```python
from build123d import *

# Parameters (mm, degrees)
DODANIE_WYCI_GNI_CIE1_DEPTH = 28
SZKIC2_R                    = 3
DODANIE_WYCI_GNI_CIE2_DEPTH = 6
DODANIE_WYCI_GNI_CIE3_DEPTH = 18


with BuildPart() as part:
    # Szkic1 → Dodanie-wyciągnięcie1 (new body)
    with BuildSketch(Plane.XY):
        Polygon((0, 0), (78, 0), (78, 46.489374011), (71.441538648, 49.547634765), (56.227281226, 16.920554432), (51.695742291, 19.033645741), (66.909999713, 51.660726074), (53.315382908, 58), (30, 8), (0, 8), align=None)
    extrude(amount=DODANIE_WYCI_GNI_CIE1_DEPTH)

    # Szkic2 → Dodanie-wyciągnięcie2 (add)
    with BuildSketch(Plane(origin=(31.737746535, 68.061817086, 0), x_dir=(0.9063077870366479, -0.4226182617407039, 0), z_dir=(0.4226182617407039, 0.906307787036648, 0))):
        with Locations((31.308287517, -7)):
            Circle(SZKIC2_R)
        with Locations((31.308287517, -21)):
            Circle(SZKIC2_R)
    extrude(amount=DODANIE_WYCI_GNI_CIE2_DEPTH)

    # Szkic3 → Dodanie-wyciągnięcie3 (add)
    with BuildSketch(Plane.XY):
        Polygon((0, 8), (0, 16), (24, 16), (24, 34), (42.123999112, 34), (30, 8), align=None)
    extrude(amount=DODANIE_WYCI_GNI_CIE3_DEPTH)


solid = part.part
```
Build history of the part. All positions in model axes, mm. A direction names the side the tool comes from. Round coordinates to 2 decimals unless told otherwise and drop trailing zeros. Loops run counter-clockwise (first coordinate to the right, second up) from the corner with the lowest first, then second, coordinate; pieces in that order, holes last.
Item 1: Two-plate mould, pull along X, no slides. Class faces 1 (the face through (62.61, 60.286, 20.958)), 2 (the face through (24, 25, 9)), 3 (the face through (59.359, 58.446, 4.972)): released by +X, released by -X, zero draft, split by the parting line, or undercut.
Item 2: Pin check, flat tips, straight feed: P1, Ø12, axis at y = 42.5, z = 6, coming from the -X side; P2, Ø1, axis at x = 47, z = 10.5, coming from the +Y side; P3, Ø5, axis at y = 34.5, z = 21, coming from the -X side. Stop position of each tip, or through.
Item 3: Which spindle directions (+Z, -Z, +X, -X, +Y, -Y) get a long thin tool onto all of the face, cutting with end or side? Do faces 4 (the face through (63.94, 33.46, 13.8)), 5 (the face through (48, 23, 0)), 6 (the face through (26, 18, 18)), 7 (the face through (33, 34, 9)). Say none if no direction does.
Item 4: Saw through at B-B (z = 11). List the corners of the cut face in (x, y), then the cut area to 3 significant figures.
Item 5: Saw through at A-A (y = 22.5). List the corners of the cut face in (x, z).
Item 6: Saw through at C-C (x = 23). List the corners of the cut face in (y, z).
Item 7: Drill centre lines: line 1 along Z through (x, y) = (30, 20); line 2 along Y through (x, z) = (23, 13); line 3 along Y through (x, z) = (12, 22.75). Where is each one in solid material? Low to high.
Item 8: Saw through at D-D (y = 13.5). List the corners of the cut face in (x, z), then the cut area to 3 significant figures.
Worked answers:
1. face 1: released by +X
1. face 2: released by -X
1. face 3: undercut
2. P1: stops at x = 43.29
2. P2: stops at y = 45.53
2. P3: stops at x = 41.19
3. face 4: +Z, -Z
3. face 5: -Z, +X, -X, +Y, -Y
3. face 6: +Z, -X, +Y
3. face 7: +Z, -Z, -X, +Y
4. outline: (0, 0) - (78, 0) - (78, 46.49) - (71.44, 49.55) - (56.23, 16.92) - (51.7, 19.03) - (66.91, 51.66) - (53.32, 58) - (42.12, 34) - (24, 34) - (24, 16) - (0, 16) - close
4. area: 2,620 mm2
5. outline: (24, 0) - (53.31, 0) - (53.31, 28) - (36.76, 28) - (36.76, 18) - (24, 18) - close; (58.83, 0) - (78, 0) - (78, 28) - (58.83, 28) - close
6. outline: (0, 0) - (16, 0) - (16, 18) - (8, 18) - (8, 28) - (0, 28) - close
7. line 1: z = 0 to 18
7. line 2: y = 0 to 16
7. line 3: y = 0 to 8
8. outline: (0, 0) - (78, 0) - (78, 28) - (32.56, 28) - (32.56, 18) - (0, 18) - close
8. area: 1,860 mm2
